```python
from build123d import *

# Parameters (mm, degrees)
SKETCH_1_R          = 2.5
SKETCH_1_R_2        = 1.5
EXTRUDE_1_DEPTH     = 10
SKETCH_2_W          = 4
SKETCH_2_H          = 4
EXTRUDE_2_DEPTH     = 3
SKETCH_3_W          = 2
SKETCH_3_H          = 0.6
CUT_EXTRUDE_1_DEPTH = 12.683321446


with BuildPart() as part:
    # 草图1 → 凸台-拉伸1 (new body)
    with BuildSketch(Plane.XY):
        Circle(SKETCH_1_R)
        Circle(SKETCH_1_R_2, mode=Mode.SUBTRACT)
    extrude(amount=EXTRUDE_1_DEPTH)

    # 草图2 → 凸台-拉伸2 (add)
    with BuildSketch(Plane(origin=(0, 0, 0), x_dir=(-1, 0, 0), z_dir=(0, 0, -1))):
        with Locations((-3.5, 0)):
            Rectangle(SKETCH_2_W, SKETCH_2_H)
    extrude(amount=-EXTRUDE_2_DEPTH)

    # 草图3 → 切除-拉伸1 (cut, through all)
    with BuildSketch(Plane(origin=(0, 0, 0), x_dir=(-1, 0, 0), z_dir=(0, 0, -1))):
        with Locations((-3, -1.7)):
            Rectangle(SKETCH_3_W, SKETCH_3_H)
        with Locations((-3, 1.7)):
            Rectangle(SKETCH_3_W, SKETCH_3_H)
    extrude(amount=-CUT_EXTRUDE_1_DEPTH, mode=Mode.SUBTRACT)


solid = part.part
```
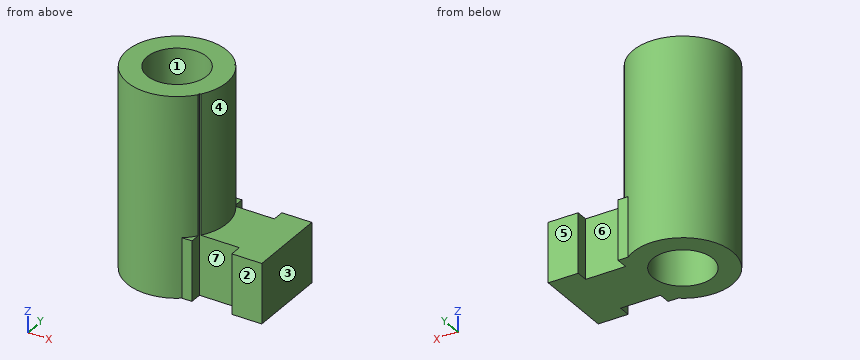
Read the model definition and answer for the solid it produces. Units are mm, in the model's axes. Face numbers are marked on the shaded views. A direction names the side the tool comes from. Give positions to 0.01 mm unless a question says otherwise; leave off trailing zeros. Write each loop counter-clockwise with the first axis right and the second up, starting at its lowest first coordinate (ties: lowest second). Pieces come first, ordered by that corner, then holes. Notation, with made-up numbers: (7, 11) - (64, 11) arc R21 ccw to (64, 20) - close; hole circle Ø4 at (62, 68.25). An arc over 180 degrees is marked (long way). Write item = value, one per line. Start each with the question number.
Item 1: Find the intervals of material crossed by probe 1 along Y at (x, z) = (0, 5.5); probe 2 along Y at (x, z) = (-0.5, 4.75), in increasing order. Write a range as [from, to].
Item 2: Find section D-D (z = 2.75). Give the vertices of the cut face in (x, y).
Item 3: Find section A-A (z = 6.5). Give the vertices of the cut face in (x, y).
Item 4: Find section C-C (y = 0). Give the vertices of the cut face in (x, z).
Item 5: The mould has two halves that part along Y. Classify the marked faces 1, 2, 3 and 4: +Y half, -Y half, draft (parallel to the pull), parting line (faces both ways), or undercut.
Item 6: A tool of negligible diameter and unlimited length cuts with its end or side. For the marked faces 5, 6 and 7, from which of +Z, -Z, +X, -X, +Y, -Y can it reach the whole face along a straight path? Write none if from no direction.
Item 7: Find section B-B (x = 0). Give the vertices of the cut face in (y, z).
Item 8: Each of these flat-tipped pins is pushed along its axis until it touches: P1, Ø1.2, axis at x = 4.5, z = 1.5, coming from the -Y side; P2, Ø0.7, axis at y = 1.5, z = 1.5, coming from the -X side; P3, Ø2.5, axis at x = 4, y = -0.5, coming from the +Z side; P4, Ø2, axis at x = 0.5, z = 3.5, coming from the -Y side. Where does it stop, or does it pass through?
Response:
q1.probe_1 = [-2.5, -1.5], [1.5, 2.5]
q1.probe_2 = [-2.45, -1.41], [1.41, 2.45]
q2.outline = (1.5, -2) - (2, -2) - (2, -1.4) - (4, -1.4) - (4, -2) - (5.5, -2) - (5.5, 2) - (4, 2) - (4, 1.4) - (2, 1.4) - (2, 2) - (1.5, 2) arc R2.5 ccw (long way) to start; hole circle Ø3 at (0, 0)
q3.outline = (2, -1.5) - (2, -1.4) - (2.07, -1.4) arc R2.5 ccw to (2.07, 1.4) - (2, 1.4) - (2, 1.5) arc R2.5 ccw (long way) to start; hole circle Ø3 at (0, 0)
q4.outline = (-2.5, 0) - (-1.5, 0) - (-1.5, 10) - (-2.5, 10) - close; (1.5, 0) - (5.5, 0) - (5.5, 3) - (2.5, 3) - (2.5, 10) - (1.5, 10) - close
q5.face_1 = undercut
q5.face_2 = -Y half
q5.face_3 = draft
q5.face_4 = parting line
q6.face_5 = +Z, -Z, +X, +Y
q6.face_6 = +Z, -Z, +Y
q6.face_7 = +Z, -Z, -Y
q7.outline = (-2.5, 0) - (-1.5, 0) - (-1.5, 10) - (-2.5, 10) - close; (1.5, 0) - (2.5, 0) - (2.5, 10) - (1.5, 10) - close
q8.P1 = -2
q8.P2 = -2.22
q8.P3 = 3
q8.P4 = -2.5
